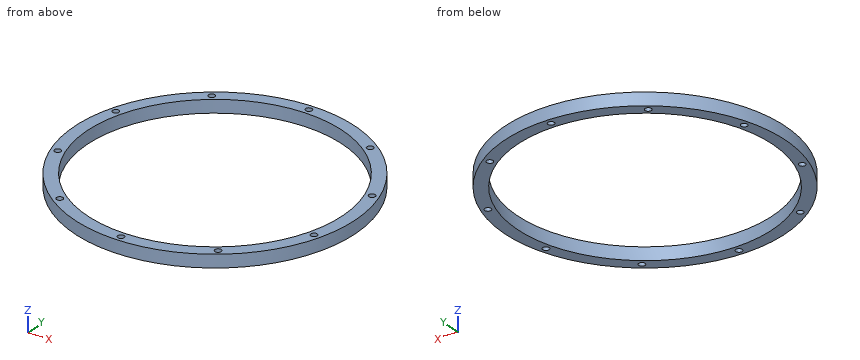
from build123d import *

# Parameters (mm, degrees)
SKETCH_1_R               = 128.7
SKETCH_1_R_2             = 117
EXTRUDE_2_DEPTH          = 11.7
SKETCH_2_R               = 2.925
CUT_EXTRUDE_2_DEPTH      = 183.384950037
PATTERN_CIRCULAR_1_COUNT = 10


with BuildPart() as part:
    # Эскиз1 → Бобышка-Вытянуть2 (new body)
    with BuildSketch(Plane.XY):
        Circle(SKETCH_1_R)
        Circle(SKETCH_1_R_2, mode=Mode.SUBTRACT)
    extrude(amount=-EXTRUDE_2_DEPTH)

    # Эскиз2 → Вырез-Вытянуть2 (cut, through all)
    with BuildSketch(Plane.XY):
        with Locations((0, 122.85)):
            Circle(SKETCH_2_R)
    cut_extrude_2 = extrude(amount=-CUT_EXTRUDE_2_DEPTH, mode=Mode.SUBTRACT)

    # Круговой массив1: Вырез-Вытянуть2 ×10 about axis
    pattern_circular_1_axis = Axis((0, 0, 0), (0, 0, 1))
    for i in range(1, PATTERN_CIRCULAR_1_COUNT):
        add(cut_extrude_2.rotate(pattern_circular_1_axis, i * 360 / PATTERN_CIRCULAR_1_COUNT), mode=Mode.SUBTRACT)


solid = part.part
Work out the finished part from the listing and answer in its coordinate system (mm). Give positions to 0.01 mm unless a question says otherwise; leave off trailing zeros. Order: outer loops, then holes, each group sorted by start corner. A loop starts at its lowest first (then second) coordinate and runs counter-clockwise, first axis right, second up. Notation, with made-up numbers: M 72,86.25 L 85,86.25 A32 cw 85,121.25 Z; hole C 4.5,34 d6. An arc over 180 degrees is marked long. Return JSON: item names as keys, results as strings.
Q1. Find the intervals of material crossed by line 1 along Y through (x, z) = (0, -2.75) (3 decimals); line 2 along X through (y, z) = (102, -8.75); line 3 along X through (y, z) = (101.5, -1.75), in increasing order. Write a range as [from, to].
Answer below:
{"line 1": "y = [-128.7, -125.775], [-119.925, -117], [117, 119.925], [125.775, 128.7]", "line 2": "x = [-78.48, -73.53], [-70.89, -57.31], [57.31, 70.89], [73.53, 78.48]", "line 3": "x = [-79.13, -74.23], [-70.19, -58.2], [58.2, 70.19], [74.23, 79.13]"}
Q2. Find section B-B, the plane y = 0. Write down the section's boundary in (x, z), and give its area (3 significant figures).
Answer below:
{"outline": "M -128.7,-11.7 L -117,-11.7 L -117,0 L -128.7,0 Z; M 117,-11.7 L 128.7,-11.7 L 128.7,0 L 117,0 Z", "area": "274 mm^2"}
Q3. Find section C-C, the plane z = -3.5. State how many separate pieces and enclosed holes the cut face has, and give its area (3 significant figures).
Answer below:
{"separate pieces": "1", "enclosed holes": "11", "area": "8,760 mm^2"}
Q4. Find section A-A, the plane x = 0. Write down the section's boundary in (y, z) (3 decimals), and give its area (3 significant figures).
Answer below:
{"outline": "M -128.7,-11.7 L -125.775,-11.7 L -125.775,0 L -128.7,0 Z; M -119.925,-11.7 L -117,-11.7 L -117,0 L -119.925,0 Z; M 117,-11.7 L 119.925,-11.7 L 119.925,0 L 117,0 Z; M 125.775,-11.7 L 128.7,-11.7 L 128.7,0 L 125.775,0 Z", "area": "137 mm^2"}
Q5. Each of these flat-tipped pins is pushed along its axis until it touches: pin 1 (1 mm diameter, centred on y = -8, z = -7.5, fed in from +X); pin 2 (1.5 mm diameter, centred on x = 11.5, z = -7, fed in from +Y); pin 3 (4.5 mm diameter, centred on x = 72.21, y = -99.39, fed in from -Z); pin 4 (4 mm diameter, centred on x = -98.5, z = -7, fed in from +Y). Where does it stop, or does it pass through?
Answer below:
{"pin 1": "stops at x = 128.48", "pin 2": "stops at y = 128.25", "pin 3": "passes through", "pin 4": "stops at y = 85.16"}
Q6. Find section D-D, the plane x = 58.5. Write down the section's boundary in (y, z).
Answer below:
{"outline": "M -114.64,-11.7 L -101.32,-11.7 L -101.32,0 L -114.64,0 Z; M 101.32,-11.7 L 114.64,-11.7 L 114.64,0 L 101.32,0 Z"}
